Model file for the job. Use its own axes, mm. A direction names the side the tool comes from. Give positions to 0.01 mm unless a question says otherwise; leave off trailing zeros. Order: outer loops, then holes, each group sorted by start corner. A loop starts at its lowest first (then second) coordinate and runs counter-clockwise, first axis right, second up. Notation, with made-up numbers: M -11.5,7.25 L 29.5,7.25 A33 ccw 29.5,42.25 Z; hole C 21,82.5 d4. An arc over 180 degrees is marked long. Return JSON: item names as keys, results as strings. Group by question number.
1. Pin check, flat tips, straight feed: pin 1 (6.5 mm diameter, centred on x = 12.7, y = 12.7, fed in from -Z); pin 2 (1 mm diameter, centred on y = 68.5, z = 2.5, fed in from +X). Stop position of each tip, or through.
2. Slice it at A-A on y = 31.75. List the corners of the cut face in (x, z) (3 decimals), then the cut area to 3 significant figures.
3. Slice it at D-D on x = 4.5. List the corners of the cut face in (y, z) (3 decimals), then the cut area to 3 significant figures.
4. Slice it at B-B on z = 1.85. Give the number of separate pieces and of enclosed holes in the cut face, then the cut area to 3 significant figures.
5. Two-plate mould, pull along X, no slides. Class faces 1 (the face through (10, 52, 0)), 2 (the face through (0, 53, 2)), 3 (the face through (27.25, 91.32, 1.57)): released by +X, released by -X, zero draft, split by the parting line, or undercut.
6. Slice it at C-C on y = 88.9. List the corners of the cut face in (x, z) (3 decimals).
7. Wall check: probe 1 along Y at (x, z) = (12.7, 0.75); probe 2 along X at (y, z) = (31.75, 2.15); probe 3 along Y at (x, z) = (10.5, 0.7). Give the ranges that are in metal, low to high. Write a range as [from, to].
8. 3-axis set-ups, long thin cutter, end or side, ignore diameter. For faces 4 (the face through (2.86, 98.88, 1.61)), 5 (the face through (25.4, 43, 2)): which of +Z, -Z, +X, -X, +Y, -Y reach the whole face in a straight line?
Autodesk Inventor part; units mm, degrees
ref_plane "YZ Plane" through (0, 0, 0) normal (1, 0, 0) x (0, 1, 0)
ref_plane "XZ Plane" through (0, 0, 0) normal (0, 1, 0) x (-1, 0, 0)
ref_plane "XY Plane" through (0, 0, 0) normal (0, 0, 1) x (1, 0, 0)
sketch "Sketch1" plane through (0, 0, 0) normal (0, 0, 1) x (1, 0, 0)
  line L0 (0, 0) -> (25.4, 0)
  line L1 (25.4, 0) -> (25.4, 101.6)
  line L2 (25.4, 101.6) -> (0, 101.6)
  line L3 (0, 101.6) -> (0, 0)
  arc A0 (25.4, 76.2) -> (25.4, 101.6) centre (25.4, 88.9) ccw
  dimension "d0" = 101.6
  dimension "d1" = 25.4
  dimension "d2" = 25.4
extrude "Extrusion1" add sketch "Sketch1" along normal blind 3.175
sketch "Sketch3" plane through (0, 0, 3.175) normal (0, 0, 1) x (1, 0, 0)
  line L0 (0, 101.6) -> (0, 0)
  line L1 (0, 0) -> (25.4, 0)
  line L2 (25.4, 101.6) -> (0, 101.6)
  line L3 (25.4, 0) -> (25.4, 76.2)
  line L4 (0, 0) -> (25.4, 0)
  line L5 (25.4, 0) -> (25.4, 63.5)
  line L6 (25.4, 63.5) -> (0, 63.5)
  line L7 (0, 63.5) -> (0, 0)
  point P0 (12.7, 50.8)
  point P1 (12.7, 12.7)
  point P2 (12.7, 31.75)
  point P3 (12.7, 0)
  dimension "d50" = 12.7
  dimension "d53" = 38.1
  dimension "d54" = 63.5
  dimension "d55" = 19.05
hole "Hole1" at (12.7, 50.8, 3.175) at (12.7, 12.7, 3.175) at (12.7, 31.75, 3.175) direction (0, 0, -1) diameter 4.8514 end through all
sketch "Sketch4" plane through (0, 0, 3.175) normal (0, 0, 1) x (1, 0, 0)
  line L0 (25.4, 0) -> (25.4, 76.2)
  arc A0 (25.4, 76.2) -> (25.4, 101.6) centre (25.4, 88.9) ccw
  point P0 (0, 0)
hole "Hole2" at (25.4, 88.9, 3.175) direction (0, 0, -1) diameter 6.096 end through all
fillet "Fillet1" radius 9.525 1 edges at (0, 101.6, 1.5875)
fillet "Fillet2" radius 1.5875 1 edges at (25.4, 76.2, 1.5875)
fillet "Fillet3" radius 12.7 2 edges at (25.4, 0, 1.5875) (0, 0, 1.5875)
equation "\"d2\" = d1"
properties part number "CLB_027_LifterBracket.ipt" material "Aluminum 6061"
Result:
{
 "1": {"pin 1": "stops at z = 0", "pin 2": "stops at x = 25.4"},
 "2": {"outline": "M 0,0 L 10.274,0 L 10.274,3.175 L 0,3.175 Z; M 15.126,0 L 25.4,0 L 25.4,3.175 L 15.126,3.175 Z", "area": "65.2 mm2"},
 "3": {"outline": "M 3.002,0 L 100.167,0 L 100.167,3.175 L 3.002,3.175 Z", "area": "308 mm2"},
 "4": {"separate pieces": "1", "enclosed holes": "4", "area": "2,660 mm2"},
 "5": {"face 1": "zero draft", "face 2": "released by -X", "face 3": "undercut"},
 "6": {"outline": "M 0,0 L 22.352,0 L 22.352,3.175 L 0,3.175 Z; M 28.448,0 L 38.1,0 L 38.1,3.175 L 28.448,3.175 Z"},
 "7": {"probe 1": "y = [0, 10.27], [15.13, 29.32], [34.18, 48.37], [53.23, 101.6]", "probe 2": "x = [0, 10.27], [15.13, 25.4]", "probe 3": "y = [0.19, 11.68], [13.72, 30.73], [32.77, 49.78], [51.82, 101.6]"},
 "8": {"face 4": "+Z, -Z, -X, +Y", "face 5": "+Z, -Z, +X, -Y"}
}
